Input: part model. Units: mm. Frame: model coordinates. A direction names the side the tool comes from. Give positions to 0.01 mm unless a question says otherwise; leave off trailing zeros. Loops run counter-clockwise (first coordinate to the right, second up) from the corner with the lowest first, then second, coordinate; pieces in that order, holes last.
from build123d import *

# Parameters (mm, degrees)
F0_W      = 76.2
F0_H      = 20.32
F0_W_2    = 55.88
F1_DEPTH  = 25
F2_T      = -2.5
F3_W      = 134.58
F3_H      = 20.32
F4_DEPTH  = 22.5
F5_T      = -2.5
F6_W      = 48.3
F6_H      = 76.2
F7_DEPTH  = 25
F8_T      = -2.5
F10_DEPTH = 30


# Not quite as in the source:
# - a shell that OpenCascade refuses in one call is made with other operations: the cavity is built on its own and cut out


with BuildPart() as f1:
    # F0 (on Top) → F1 (new body)
    with BuildSketch(Plane.XY):
        Polygon((-361.3686263561, 74.1551402664), (-361.3686263561, 48.7551402664), (-285.1686263561, 48.7551402664), (-229.2886263561, 48.7551402664), (-178.4886263561, 48.7551402664), (-178.4886263561, -27.4448597336), (-148.0086263561, -27.4448597336), (-148.0086263561, 150.3551402664), (-236.9086263561, 150.3551402664), (-272.4686263561, 150.3551402664), (-361.3686263561, 150.3551402664), align=None)
        with Locations((-323.2686263561, 38.5951402664)):
            Rectangle(F0_W, F0_H)
        with Locations((-257.2286263561, 38.5951402664)):
            Rectangle(F0_W_2, F0_H)
        Polygon((-178.4886263561, 48.7551402664), (-229.2886263561, 48.7551402664), (-229.2886263561, 28.4351402664), (-229.2886263561, -27.4448597336), (-178.4886263561, -27.4448597336), align=None)
        Polygon((-178.4886263561, -27.4448597336), (-229.2886263561, -27.4448597336), (-229.2886263561, -121.4248597336), (-127.6886263561, -121.4248597336), (-127.6886263561, 150.3551402664), (-148.0086263561, 150.3551402664), (-148.0086263561, -27.4448597336), align=None)
    extrude(amount=F1_DEPTH)

    # F2
    f2_openings = [f1.faces().sort_by_distance(p)[0] for p in [
        (-221.527682, 42.066274, 25),
    ]]
    offset(amount=F2_T, openings=f2_openings, kind=Kind.INTERSECTION)

    # F3 (on face) → F4 (join)
    with BuildSketch(Plane.XY.offset(2.5)):
        with Locations((-294.0786263561, 38.5951402664)):
            Rectangle(F3_W, F3_H)
    extrude(amount=F4_DEPTH)

    # F5: a shell. OpenCascade refuses it in one call, so the cavity is built on its own and cut out:
    # the body offset inwards by the wall thickness, plus a prism from it out through each open face.
    f5_core = offset(f1.part, amount=F5_T, kind=Kind.INTERSECTION, mode=Mode.PRIVATE)
    f5_exits = [f5_core.faces().sort_by_distance(p)[0] for p in [
        (-294.078626, 38.59514, 22.5),
    ]]
    add(f5_core, mode=Mode.SUBTRACT)
    extrude(f5_exits, amount=-F5_T, mode=Mode.SUBTRACT)

    # F6 (on Top) → F7 (join)
    with BuildSketch(Plane.XY):
        with Locations((-202.6386263561, 10.6551402664)):
            Rectangle(F6_W, F6_H)
    extrude(amount=F7_DEPTH)

    # F8: a shell. OpenCascade refuses it in one call, so the cavity is built on its own and cut out:
    # the body offset inwards by the wall thickness, plus a prism from it out through each open face.
    f8_core = offset(f1.part, amount=F8_T, kind=Kind.INTERSECTION, mode=Mode.PRIVATE)
    f8_exits = [f8_core.faces().sort_by_distance(p)[0] for p in [
        (-203.888626, 10.65514, 22.5),
    ]]
    add(f8_core, mode=Mode.SUBTRACT)
    extrude(f8_exits, amount=-F8_T, mode=Mode.SUBTRACT)

    # F9 (on Top) → F10 (cut)
    with BuildSketch(Plane.XY):
        Polygon((-358.8686263561, 60.7551402664), (-361.3686263561, 60.7551402664), (-361.3686263561, 51.7551402664), (-358.8686263561, 50.7551402664), align=None)
    extrude(amount=F10_DEPTH, mode=Mode.SUBTRACT)


solid = f1.part
(1) Cut plane C-C (x = -205). Return the cut outline in (y, z).
Values follow:
outline: (-121.42, 0) - (150.36, 0) - (150.36, 25) - (147.86, 25) - (147.86, 2.5) - (48.76, 2.5) - (48.76, 25) - (46.26, 25) - (46.26, 2.5) - (-24.94, 2.5) - (-24.94, 25) - (-27.44, 25) - (-27.44, 2.5) - (-118.92, 2.5) - (-118.92, 25) - (-121.42, 25) - close
(2) Reachability of faces 4 (the flat face through (-293, 46.255, 14)), 5 (the flat face through (-243, 150.355, 12)) from +Z, -Z, +X, -X, +Y, -Y: full face, straight path, thin tool, end or side. Return the list, or none.
Values follow:
face 4: +Z
face 5: +Z, -Z, +X, -X, +Y
(3) Mould query, pull axis X, two halves, no side actions, for faces 1 (the flat face through (-361.369, 40, 12)), 2 (the flat face through (-295, 39, 2.5)), 3 (the flat face through (-220, 47, 0)). Classes: +X half, -X half, draft (parallel to the pull), parting line (faces both ways), or undercut.
Values follow:
face 1: -X half
face 2: undercut
face 3: draft
(4) Cut plane B-B (y = -97.5). Return the cut outline in (x, z).
Values follow:
outline: (-229.29, 0) - (-127.69, 0) - (-127.69, 25) - (-130.19, 25) - (-130.19, 2.5) - (-226.79, 2.5) - (-226.79, 25) - (-229.29, 25) - close
(5) Cut plane D-D (y = 1). Return the cut outline in (x, z).
Values follow:
outline: (-229.29, 0) - (-127.69, 0) - (-127.69, 25) - (-130.19, 25) - (-130.19, 2.5) - (-178.49, 2.5) - (-178.49, 25) - (-180.99, 25) - (-180.99, 2.5) - (-226.79, 2.5) - (-226.79, 25) - (-229.29, 25) - close
(6) Ray query, probe 1 along X at (y, z) = (2, 20); probe 2 along Y at (x, z) = (-262, 20.25); probe 3 along Y at (x, z) = (-194, 21). Return the intervals inside material, ascending.
Values follow:
probe 1: x = -229.29 to -226.79, -180.99 to -178.49, -130.19 to -127.69
probe 2: y = 28.44 to 30.94, 46.26 to 48.76, 147.86 to 150.36
probe 3: y = -121.42 to -118.92, -27.44 to -24.94, 46.26 to 48.76, 147.86 to 150.36
(7) Cut plane A-A (z = 7.75). Return the cut outline in (x, y).
Values follow:
outline: (-361.37, 28.44) - (-229.29, 28.44) - (-229.29, -121.42) - (-127.69, -121.42) - (-127.69, 150.36) - (-361.37, 150.36) - (-361.37, 60.76) - (-358.87, 60.76) - (-358.87, 147.86) - (-130.19, 147.86) - (-130.19, -118.92) - (-226.79, -118.92) - (-226.79, -27.44) - (-178.49, -27.44) - (-178.49, 48.76) - (-358.87, 48.76) - (-358.87, 50.76) - (-361.37, 51.76) - close; hole (-358.87, 30.94) - (-229.29, 30.94) - (-229.29, 46.26) - (-358.87, 46.26) - close; hole (-226.79, -24.94) - (-180.99, -24.94) - (-180.99, 46.26) - (-226.79, 46.26) - close
(8) Pin query (flat end, axial travel): pin 1 Ø1.5 at (y, z) = (-68, 3.5) entering from -X; pin 2 Ø13.5 at (x, y) = (-215, 20.5) entering from +Z; pin 3 Ø3 at (y, z) = (56, 1) entering from -X. Return the tip coordinate at first contact, or that it passes through.
Values follow:
pin 1: stops at x = -229.29
pin 2: stops at z = 2.5
pin 3: stops at x = -358.87
